For this review, use the dimensioned drawing (mm, ordinates from the lowest corner) and the shaded views. A direction names the side the tool comes from. Give positions to 0.01 mm unless a question says otherwise; leave off trailing zeros. Order: outer loops, then holes, each group sorted by start corner. A loop starts at its lowest first (then second) coordinate and runs counter-clockwise, first axis right, second up. Notation, with made-up numbers: (-35, -37) -> (-9, -37) arc R34 ccw to (-9, -7) -> close; hole circle Ø11 at (-39.5, 21). An arc over 180 degrees is marked (long way). Answer as a JSON object with one key per item and string values. Group by question number.
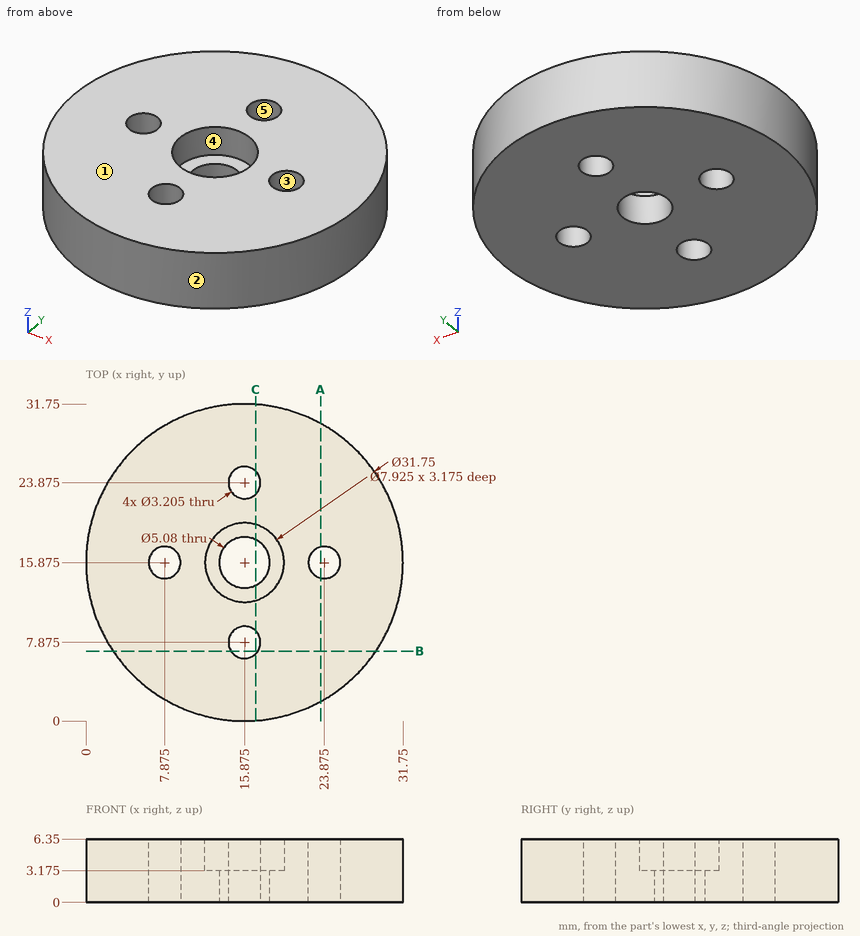
1. Take a section at C-C on x = 17. State how many separate pieces and enclosed holes the cut face has.
2. Take a section at B-B on y = 7. Give the boundary of the cut face in (x, z).
3. Draft analysis for pull direction X (two halves, no side actions). For the marked faces 1, 2 and 3, state which applies: pulls with the +X half, pulls with the -X half, needs draft (parallel to the pull), parting line crosses it, or undercut.
4. For pin 1 (4 mm diameter, centred on x = 16, y = 16.5, fed in from +Z) (3 decimals), flat-tipped, find the tip position at first contact; note if it passes through.
5. Take a section at A-A on x = 23.5. Give the boundary of the cut face in (y, z).
6. For probe 1 along X at (y, z) = (14.5, 2); probe 2 along Y at (x, z) = (16.5, 5.75); probe 3 along X at (y, z) = (15, 4.25) (1 decimal), list the stretches that pass through material, from the lowest coordinate up. Write a range as [from, to].
7. Machinability: for the marked faces 4 and 5, which of the approach directions +Z, -Z, +X, -X, +Y, -Y give a long, thin tool a straight path to every point of the face, cutting with its end or side? Answer none if there is none.
Checks:
{
 "1": {"separate pieces": "4", "enclosed holes": "0"},
 "2": {"outline": "(2.71, 0) -> (14.53, 0) -> (14.53, 6.35) -> (2.71, 6.35) -> close; (17.22, 0) -> (29.04, 0) -> (29.04, 6.35) -> (17.22, 6.35) -> close"},
 "3": {"face 1": "needs draft", "face 2": "parting line crosses it", "face 3": "undercut"},
 "4": {"pin 1": "stops at z = 3.175"},
 "5": {"outline": "(1.95, 0) -> (14.32, 0) -> (14.32, 6.35) -> (1.95, 6.35) -> close; (17.43, 0) -> (29.8, 0) -> (29.8, 6.35) -> (17.43, 6.35) -> close"},
 "6": {"probe 1": "x = [0.06, 7.05], [8.7, 13.74], [18.01, 23.05], [24.7, 31.69]", "probe 2": "y = [0.01, 6.4], [9.35, 11.96], [19.79, 22.4], [25.35, 31.74]", "probe 3": "x = [0, 6.5], [9.2, 12], [19.7, 22.5], [25.2, 31.7]"},
 "7": {"face 4": "+Z", "face 5": "+Z, -Z"}
}
